Autodesk Inventor part; units mm, degrees
ref_plane "YZ Plane" through (0, 0, 0) normal (1, 0, 0) x (0, 1, 0)
ref_plane "XZ Plane" through (0, 0, 0) normal (0, 1, 0) x (-1, 0, 0)
ref_plane "XY Plane" through (0, 0, 0) normal (0, 0, 1) x (1, 0, 0)
sketch "Sketch1" plane through (0, 0, 0) normal (0, 1, 0) x (-1, 0, 0)
  circle A0 centre (50, 0) radius 1.75
  circle A1 centre (35.016, -56.1406) radius 1.75
  line L0 (0, 113.2764) -> (0, -120.1992) construction
  line L1 (64.7812, 0) -> (-65.3256, 0) construction
  ellipse E0 centre (0, 0) end of major axis (-50, 0) minor radius 78.647 construction
  circle A2 centre (-50, 0) radius 1.75
  circle A3 centre (-35.016, -56.1406) radius 1.75
  circle A4 centre (35.016, 56.1406) radius 1.75
  circle A5 centre (-35.016, 56.1406) radius 1.75
  ellipse E1 centre (0, 0) end of major axis (-0.2534, -85.9996) minor radius 56
  circle A6 centre (10.5, 32.5) radius 1
  circle A7 centre (10.5, 20) radius 1
  circle A8 centre (-10.5, 32.5) radius 1
  circle A9 centre (-10.5, 20) radius 1
  circle A10 centre (14, -30) radius 1
  circle A11 centre (-14, -30) radius 1
  line L2 (12, -18) -> (-12, -18)
  line L3 (-12, -18) -> (-12, -42)
  line L4 (-12, -42) -> (12, -42)
  line L5 (12, -42) -> (12, -18)
  line L6 (-4.25, 24.25) -> (4.25, 24.25)
  line L7 (4.25, 24.25) -> (4.25, 15.75)
  line L8 (4.25, 15.75) -> (-4.25, 15.75)
  line L9 (-4.25, 15.75) -> (-4.25, 24.25)
  dimension "d55" = 78.647
  dimension "d56" = 50
  dimension "d60" = 86
  dimension "d61" = 56
  dimension "d49" = 3.5
  dimension "d58" = 3.5
  dimension "d59" = 35.016
  dimension "d66" = 2
  dimension "d69" = 12.5
  dimension "d72" = 21
  dimension "d75" = 10.5
  dimension "d76" = 20
  dimension "d77" = 2
  dimension "d78" = 28
  dimension "d79" = 30
  dimension "d80" = 24
  dimension "d81" = 24
  dimension "d82" = 12
  dimension "d83" = 12
  dimension "d84" = 8.5
  dimension "d85" = 8.5
  dimension "d86" = 4.25
  dimension "d87" = 4.25
extrude "Extrusion7" add sketch "Sketch1" along normal blind 3
properties part number "TopCover"
Input: part model. Units: mm. Frame: model coordinates. Give positions to 0.01 mm unless a question says otherwise; leave off trailing zeros.
1. Mould query, pull axis Z, two halves, no side actions, for faces 1 (the cylindrical face through (34.08, 1.48, 54.66)), 2 (the flat face through (1, 0, 1)). Classes: released by +Z, released by -Z, zero draft, split by the parting line, or undercut.
Derived:
face 1: undercut
face 2: zero draft
2. Section A-A on z = 0. Give the number of separate pieces and of enclosed holes in the cut face, and give its area (3 significant figures).
Derived:
separate pieces: 3
enclosed holes: 0
area: 315 mm2
3. Material intervals for L1, parallel to Z at x = -34.5, y = 1.5; L2, parallel to X at y = 0.3, z = -1; L3, parallel to X at y = 2.3, z = -57.5, sorted ascending.
Derived:
L1: z = -67.6 to -57.81, -54.47 to 54.47, 57.81 to 67.88
L2: x = -55.99 to -51.44, -48.56 to 48.56, 51.44 to 56
L3: x = -41.55 to -36.12, -33.91 to 33.91, 36.12 to 41.74
4. Pin query (flat end, axial travel): pin 1 (0.9 mm diameter, centred on y = 1.5, z = 19, fed in from -X); pin 2 (1.5 mm diameter, centred on y = 2, z = -33, fed in from -X); pin 3 (1 mm diameter, centred on x = 41, y = 1, fed in from +Z). Return the tip coordinate at first contact, or that it passes through.
Derived:
pin 1: stops at x = -54.71
pin 2: stops at x = -51.86
pin 3: stops at z = 59.23
